from build123d import *

# Parameters (mm, degrees)
F0_W      = 11.5
F0_H      = 6
F1_DEPTH  = 15
F2_W      = 11.3
F2_H      = 11.3
F3_DEPTH  = 24
F5_W      = 12.6701932168
F5_H      = 0.4
F6_DEPTH  = 5.5
F7_W      = 9.9
F7_H      = 0.3
F8_DEPTH  = 6
F9_D      = 4.9
F10_DEPTH = 4


with BuildPart() as f1:
    # F0 (on Front) → F1 (new body)
    with BuildSketch(Plane.XZ):
        with BuildLine():
            ThreePointArc((11.5, 6), (5.75, 11.75), (0, 6))
            Line((0, 6), (11.5, 6))
        make_face()
        with Locations((5.75, 3)):
            Rectangle(F0_W, F0_H)
    extrude(amount=F1_DEPTH)

    # F2 (on face) → F3 (join)
    with BuildSketch(Plane.XZ.offset(15)):
        with Locations((5.75, 5.65)):
            Rectangle(F2_W, F2_H)
    extrude(amount=F3_DEPTH)

    # F5 (on 3pt) → F6 (cut)
    with BuildSketch(Plane(origin=(0, 0, 6), x_dir=(1, 0, 0), z_dir=(0, 0, -1))):
        with Locations((6.4887672779, 12.7)):
            Rectangle(F5_W, F5_H)
    extrude(amount=-F6_DEPTH, mode=Mode.SUBTRACT)

    # F7 (on face) → F8 (cut, through all)
    with BuildSketch(Plane(origin=(0, 0, 0), x_dir=(1, 0, 0), z_dir=(0, 0, -1))):
        with Locations((5.75, 12.7)):
            Rectangle(F7_W, F7_H)
    extrude(amount=-F8_DEPTH, mode=Mode.SUBTRACT)

    # F9 (through all)
    with Locations(Plane(origin=(0, 0, 0), x_dir=(1, 0, 0), z_dir=(0, 0, -1))):
        with Locations((5.65, 29)):
            Hole(F9_D / 2)

    # F5 (on 3pt) → F10 (cut)
    with BuildSketch(Plane(origin=(0, 0, 6), x_dir=(1, 0, 0), z_dir=(0, 0, -1))):
        with Locations((6.4887672779, 12.7)):
            Rectangle(F5_W, F5_H)
    extrude(amount=F10_DEPTH, mode=Mode.SUBTRACT)


solid = f1.part
The listing builds one solid part. Answer for the finished solid, in the listing's coordinates (mm). A direction names the side the tool comes from. Round coordinates to 2 decimals unless told otherwise and drop trailing zeros. Write each loop counter-clockwise with the first axis right and the second up, starting at its lowest first coordinate (ties: lowest second). Pieces come first, ordered by that corner, then holes. Notation, with made-up numbers: (0, 58.25) - (28, 58.25) arc R23 ccw to (28, 92.25) - close; hole circle Ø7 at (33, 55). An arc over 180 degrees is marked (long way). Use a Markdown table: item, result. Add a question column.
1. Consider line 1 (Y direction, x = 5.65, z = 3.5); line 2 (X direction, y = -29, z = 8.75); line 3 (Y direction, x = 6.5, z = 4.75). Determine where each line is inside the solid, lowest interval first.
2. The part is cut by section B-B (y = -29). Write down the section's boundary in (x, z).
3. The part is cut by section D-D (y = -5.5). Write down the section's boundary in (x, z), and give its area (3 significant figures).
4. The part is cut by section A-A (x = 5.65). Write down the section's boundary in (y, z), and give its area (3 significant figures).
5. The part is cut by section C-C (x = 2). Write down the section's boundary in (y, z).
6. For a pull along Y with two mould halves and no side action, classify faces 1 (the face through (6, -39, 6)), 2 (the face through (5.97, -31.43, 5.73)), 3 (the face through (10.4, -15, 10.3)), 4 (the face through (0, -7, 3)) as +Y half, -Y half, draft (parallel to the pull), parting line (faces both ways), or undercut.
7. A tool of negligible diameter and unlimited length cuts with its end or side. For faces 5 (the face through (11.4, -27, 6)), 6 (the face through (6, -12.5, 7)), 7 (the face through (6, -12.85, 1)), from which of +Z, -Z, +X, -X, +Y, -Y can it reach the whole face along a straight path? Write none if from no direction.
8. Flat-ended cylindrical pins translate along their axes: P1, Ø1.5, axis at x = 7, y = -24, coming from the +Z side; P2, Ø1.5, axis at y = -24, z = 5.5, coming from the -X side; P3, Ø6, axis at x = 2, z = 8.5, coming from the +Y side; P4, Ø5.5, axis at y = -28.5, z = 8, coming from the +X side. Find the tip coordinate at first contact, or state that the pin passes through.
Reported:
| question | item | result |
|---|---|---|
| 1 | line 1 | -39 to -31.45, -26.55 to -12.9, -12.5 to 0 |
| 1 | line 2 | 0.1 to 3.2, 8.1 to 11.4 |
| 1 | line 3 | -39 to -31.3, -26.7 to -12.9, -12.5 to 0 |
| 2 | outline | (0.1, 0) - (3.2, 0) - (3.2, 11.3) - (0.1, 11.3) - close; (8.1, 0) - (11.4, 0) - (11.4, 11.3) - (8.1, 11.3) - close |
| 3 | outline | (0, 0) - (11.5, 0) - (11.5, 6) arc R5.75 ccw to (0, 6) - close |
| 3 | area | 121 mm^2 |
| 4 | outline | (-39, 0) - (-31.45, 0) - (-31.45, 11.3) - (-39, 11.3) - close; (-26.55, 0) - (-12.85, 0) - (-12.85, 2) - (-12.9, 2) - (-12.9, 11.5) - (-12.5, 11.5) - (-12.5, 2) - (-12.55, 2) - (-12.55, 0) - (0, 0) - (0, 11.75) - (-15, 11.75) - (-15, 11.3) - (-26.55, 11.3) - close |
| 4 | area | 388 mm^2 |
| 5 | outline | (-39, 0) - (-12.85, 0) - (-12.85, 2) - (-12.9, 2) - (-12.9, 10.36) - (-15, 10.36) - (-15, 11.3) - (-39, 11.3) - close; (-12.55, 0) - (0, 0) - (0, 10.36) - (-12.5, 10.36) - (-12.5, 2) - (-12.55, 2) - close |
| 6 | face 1 | -Y half |
| 6 | face 2 | undercut |
| 6 | face 3 | +Y half |
| 6 | face 4 | draft |
| 7 | face 5 | +Z, -Z, +X, -Y |
| 7 | face 6 | +X |
| 7 | face 7 | -Z |
| 8 | P1 | z = 11.3 |
| 8 | P2 | x = 0.1 |
| 8 | P3 | y = 0 |
| 8 | P4 | x = 11.4 |
